Verification items for the finished model (mm, model axes). Face numbers are marked on the shaded views. A direction names the side the tool comes from. Give positions to 0.01 mm unless a question says otherwise; leave off trailing zeros. Write each loop counter-clockwise with the first axis right and the second up, starting at its lowest first coordinate (ties: lowest second). Pieces come first, ordered by that corner, then holes.
from build123d import *

# Parameters (mm, degrees)
SKETCH1_R           = 1.5
BOSS_EXTRUDE1_DEPTH = 12
SKETCH2_R           = 6.695859604
BOSS_EXTRUDE2_DEPTH = 9.4028
CUT_EXTRUDE2_DEPTH  = 64.105652153
HOLE1_D             = 5.2324
CUT_EXTRUDE3_DEPTH  = 11
SKETCH8_R           = 19.05
CUT_EXTRUDE4_DEPTH  = 10
SKETCH9_R           = 6.35
CUT_EXTRUDE6_DEPTH  = 1.27
CUT_EXTRUDE7_DEPTH  = 60.624425826


with BuildPart() as part:
    # Sketch1 → Boss-Extrude1 (new body)
    with BuildSketch(Plane.XY):
        Polygon((-40.843506262, 22.426308796), (-1, -46.5846684), (1, -46.5846684), (40.843506262, 22.426308796), (39.843506262, 24.158359604), (-39.843506262, 24.158359604), align=None)
        with Locations((-30.245937227, 17.4625)):
            Circle(SKETCH1_R, mode=Mode.SUBTRACT)
        with Locations((30.245937227, 17.4625)):
            Circle(SKETCH1_R, mode=Mode.SUBTRACT)
        with Locations((0, -34.925)):
            Circle(SKETCH1_R, mode=Mode.SUBTRACT)
    extrude(amount=BOSS_EXTRUDE1_DEPTH)

    # Sketch2 → Boss-Extrude2 (add)
    with BuildSketch(Plane(origin=(0, 0, 0), x_dir=(-1, 0, 0), z_dir=(0, 0, -1))):
        with Locations(Location((30.245937227, 17.4625, 0), (0, 0, 90))):
            Circle(SKETCH2_R)
        with Locations(Location((-30.245937227, 17.4625, 0), (0, 0, 210))):
            Circle(SKETCH2_R)
        with Locations(Location((0, -34.925, 0), (0, 0, 210))):
            Circle(SKETCH2_R)
    extrude(amount=BOSS_EXTRUDE2_DEPTH)

    # Sketch3 → Cut-Extrude2 (cut, through all)
    with BuildSketch(Plane(origin=(0, 0, 0), x_dir=(-1, 0, 0), z_dir=(0, 0, -1))):
        with BuildLine():
            Line((-5.798784517, -38.272929802), (-1, -46.5846684))
            Line((-1, -46.5846684), (1, -46.5846684))
            Line((1, -46.5846684), (5.798784517, -38.272929802))
            ThreePointArc((5.798784517, -38.272929802), (0, -41.620859604), (-5.798784517, -38.272929802))
        make_face()
        with BuildLine():
            Line((-30.245937227, 24.158359604), (-39.843506262, 24.158359604))
            Line((-39.843506262, 24.158359604), (-40.843506262, 22.426308796))
            Line((-40.843506262, 22.426308796), (-36.044721744, 14.114570198))
            ThreePointArc((-36.044721744, 14.114570198), (-36.044721744, 20.810429802), (-30.245937227, 24.158359604))
        make_face()
        with BuildLine():
            Line((36.044721744, 14.114570198), (40.843506262, 22.426308796))
            Line((40.843506262, 22.426308796), (39.843506262, 24.158359604))
            Line((39.843506262, 24.158359604), (30.245937227, 24.158359604))
            ThreePointArc((30.245937227, 24.158359604), (36.044721744, 20.810429802), (36.044721744, 14.114570198))
        make_face()
    extrude(amount=-CUT_EXTRUDE2_DEPTH, mode=Mode.SUBTRACT)

    # Hole1 (through all)
    with Locations(Plane.XY.offset(12)):
        with Locations((-30.245937227, 17.4625), (30.245937227, 17.4625), (0, -34.925)):
            Hole(HOLE1_D / 2)

    # Sketch7 → Cut-Extrude3 (cut)
    with BuildSketch(Plane.XY.offset(12)):
        with BuildLine():
            Line((-19.554402665, 21.158359604), (19.554402665, 21.158359604))
            ThreePointArc((19.554402665, 21.158359604), (22.342326137, 20.026718493), (23.552785201, 17.272100961))
            ThreePointArc((23.552785201, 17.272100961), (24.44715271, 14.114570198), (26.734470809, 11.761259834))
            ThreePointArc((26.734470809, 11.761259834), (28.514810038, 9.335662768), (28.100878252, 6.355429662))
            Line((28.100878252, 6.355429662), (8.546475587, -27.513789266))
            ThreePointArc((8.546475587, -27.513789266), (6.1724839, -29.362381261), (3.181685608, -29.033360795))
            ThreePointArc((3.181685608, -29.033360795), (0, -28.229140396), (-3.181685608, -29.033360795))
            ThreePointArc((-3.181685608, -29.033360795), (-6.1724839, -29.362381261), (-8.546475587, -27.513789266))
            Line((-8.546475587, -27.513789266), (-28.100878252, 6.355429662))
            ThreePointArc((-28.100878252, 6.355429662), (-28.514810038, 9.335662768), (-26.734470809, 11.761259834))
            ThreePointArc((-26.734470809, 11.761259834), (-24.44715271, 14.114570198), (-23.552785201, 17.272100961))
            ThreePointArc((-23.552785201, 17.272100961), (-22.342326137, 20.026718493), (-19.554402665, 21.158359604))
        make_face()
    extrude(amount=-CUT_EXTRUDE3_DEPTH, mode=Mode.SUBTRACT)

    # Sketch8 → Cut-Extrude4 (cut)
    with BuildSketch(Plane.XY.offset(1)):
        Circle(SKETCH8_R)
    extrude(amount=-CUT_EXTRUDE4_DEPTH, mode=Mode.SUBTRACT)

    # Sketch9 → Cut-Extrude6 (cut)
    with BuildSketch(Plane.XY.offset(12)):
        with BuildLine():
            Line((5.798784517, -38.272929802), (36.044721744, 14.114570198))
            ThreePointArc((36.044721744, 14.114570198), (36.044721744, 20.810429802), (30.245937227, 24.158359604))
            Line((30.245937227, 24.158359604), (-30.245937227, 24.158359604))
            ThreePointArc((-30.245937227, 24.158359604), (-36.044721744, 20.810429802), (-36.044721744, 14.114570198))
            Line((-36.044721744, 14.114570198), (-5.798784517, -38.272929802))
            ThreePointArc((-5.798784517, -38.272929802), (0, -41.620859604), (5.798784517, -38.272929802))
        make_face()
        with Locations((-30.245937227, 17.4625)):
            Circle(SKETCH9_R, mode=Mode.SUBTRACT)
        with Locations((30.245937227, 17.4625)):
            Circle(SKETCH9_R, mode=Mode.SUBTRACT)
        with Locations((0, -34.925)):
            Circle(SKETCH9_R, mode=Mode.SUBTRACT)
    extrude(amount=-CUT_EXTRUDE6_DEPTH, mode=Mode.SUBTRACT)

    # Sketch10 → Cut-Extrude7 (cut, through all)
    with BuildSketch(Plane.XY.offset(12)):
        with BuildLine():
            Line((-32.862137227, 17.4625), (-32.862137227, 23.626105552))
            ThreePointArc((-32.862137227, 23.626105552), (-31.580833929, 24.023946992), (-30.245937227, 24.158359604))
            Line((-30.245937227, 24.158359604), (-27.629737227, 24.158359604))
            Line((-27.629737227, 24.158359604), (-27.629737227, 17.4625))
            ThreePointArc((-27.629737227, 17.4625), (-30.245937227, 14.8463), (-32.862137227, 17.4625))
        make_face()
        with BuildLine():
            Line((30.245937227, 24.158359604), (27.629737227, 24.158359604))
            Line((27.629737227, 24.158359604), (27.629737227, 17.4625))
            ThreePointArc((27.629737227, 17.4625), (30.245937227, 14.8463), (32.862137227, 17.4625))
            Line((32.862137227, 17.4625), (32.862137227, 23.626105552))
            ThreePointArc((32.862137227, 23.626105552), (31.580833929, 24.023946992), (30.245937227, 24.158359604))
        make_face()
        with BuildLine():
            Line((-19.05, 0), (-19.05, 24.158359604))
            Line((-19.05, 24.158359604), (19.05, 24.158359604))
            Line((19.05, 24.158359604), (19.05, 0))
            ThreePointArc((19.05, 0), (18.113838196, -5.898420621), (15.397363169, -11.217116717))
            Line((15.397363169, -11.217116717), (2.6162, -28.761394448))
            Line((2.6162, -28.761394448), (2.6162, -34.925))
            ThreePointArc((2.6162, -34.925), (0, -37.5412), (-2.6162, -34.925))
            Line((-2.6162, -34.925), (-2.6162, -28.761394448))
            Line((-2.6162, -28.761394448), (-15.397363169, -11.217116717))
            ThreePointArc((-15.397363169, -11.217116717), (-18.113838196, -5.898420621), (-19.05, 0))
        make_face()
    extrude(amount=-CUT_EXTRUDE7_DEPTH, mode=Mode.SUBTRACT)


solid = part.part
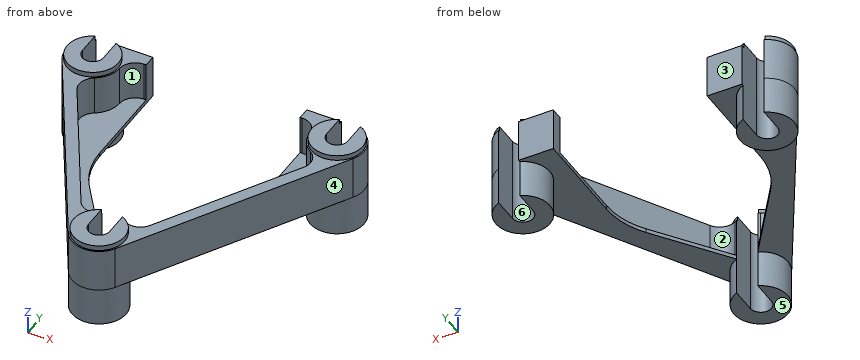
Item 1: Scan lines: line 1 along Z through (x, y) = (-16, -15); line 2 along X through (y, z) = (17, 7.75); line 3 along X through (y, z) = (-16.5, 3). Record each from-to range of solid material in increasing order.
Answer key:
line 1: z = 0 to 10.73
line 2: x = -36.93 to -32.82, -27.67 to -23.57, 23.57 to 27.67, 32.82 to 36.93
line 3: x = -18.37 to -14.91, 14.91 to 18.37
Item 2: Set-up check for the marked faces 1, 2 and 3: record each of +Z, -Z, +X, -X, +Y, -Y from which the full face is reachable in a straight line by a thin tool's end or side.
Answer key:
face 1: +Z
face 2: +Z, +Y
face 3: +Z, -Z, +X, -X, +Y
Item 3: Sectioned sample at C-C on x = 0. Record the cut outline in (y, z) (3 decimals).
Answer key:
outline: (-41.621, -9.403) - (-37.541, -9.403) - (-37.541, 12) - (-41.275, 12) - (-41.275, 10.73) - (-41.621, 10.73) - close
Item 4: Sectioned sample at D-D on x = 29.5. Record the cut outline in (y, z).
Answer key:
outline: (2.78, 0) - (10.81, 0) - (10.81, -9.4) - (14.95, -9.4) - (14.95, 12) - (11.16, 12) - (11.16, 10.73) - (2.78, 10.73) - close
Item 5: Depth check by flat-ended pin: pin 1 (0.6 mm diameter, centred on x = -19.5, z = 4, fed in from -Y); pin 2 (5 mm diameter, centred on y = -31, z = 0, fed in from -X); pin 3 (10 mm diameter, centred on x = 1, z = 8, fed in from +Y); pin 4 (3 mm diameter, centred on y = 17, z = 8, fed in from +X). Enter the tip coordinate at first touch or a pass-through.
Answer key:
pin 1: stops at y = -15.06
pin 2: stops at x = -11.44
pin 3: stops at y = -28.76
pin 4: stops at x = 36.94
Item 6: Release check for a two-part mould opening along X. For the marked faces 4, 5 and 6 record: released by +X, released by -X, zero draft, split by the parting line, or undercut.
Answer key:
face 4: released by +X
face 5: zero draft
face 6: undercut
Item 7: Sectioned sample at A-A on z = -7. Record the cut outline in (x, y) (1 decimal).
Answer key:
outline: (-32.9, 17.5) - (-32.9, 23.6) arc R6.7 ccw (long way) to (-27.6, 23.6) - (-27.6, 17.5) arc R2.6 cw to start; (-2.6, -34.9) - (-2.6, -28.8) arc R6.7 ccw (long way) to (2.6, -28.8) - (2.6, -34.9) arc R2.6 cw to start; (27.6, 17.5) - (27.6, 23.6) arc R6.7 ccw (long way) to (32.9, 23.6) - (32.9, 17.5) arc R2.6 cw to start
